Geometry check sheet. Reference: the model listing, model coordinates, mm. A direction names the side the tool comes from. Round coordinates to 2 decimals unless told otherwise and drop trailing zeros. Loops run counter-clockwise (first coordinate to the right, second up) from the corner with the lowest first, then second, coordinate; pieces in that order, holes last. Notation, with made-up numbers: (-15, -22.75) -> (36, -22.75) arc R20 ccw to (36, -2.75) -> close; hole circle Ø5 at (36.5, -26). An arc over 180 degrees is marked (long way). Use a Markdown table: item, result. Add a question column.
Q1. Gauge pin test, flat ends, axial feed: P1, Ø3, axis at y = 15, z = 1.5, coming from the -X side; P2, Ø12, axis at x = -6.5, z = 19, coming from the +Y side; P3, Ø12, axis at x = -13, z = -7, coming from the +Y side. Record the tip position at first contact, or that the pin passes through.
Q2. Material ranges on L1, parallel to X at y = 3, z = -16; L2, parallel to X at y = 3, z = -17.5; L3, parallel to Z at x = -66, y = -18, recorded low to high.
Q3. Sectioned sample at D-D, the plane x = -61.5. Enter the section's corners in (y, z).
Q4. Sectioned sample at B-B, the plane x = -71.5. Enter the section's corners in (y, z), then the cut area to 3 significant figures.
Q5. Sectioned sample at A-A, the plane z = 0. Enter the section's corners in (x, y).
Q6. Set-up check for faces 1 (the face through (-63, -22.057, 0)), 2 (the face through (-63, 14.021, 0)), 3 (the face through (-8.89, -8, -15)): record each of +Z, -Z, +X, -X, +Y, -Y from which the full face is reachable in a straight line by a thin tool's end or side.
Q7. Release check for a two-part mould opening along X. For faces 4 (the face through (-7.602, -17.576, 5.535)), 5 (the face through (-71, -18, -9.142)), 6 (the face through (-56.896, 0, -12)), 7 (the face through (-56.896, -19, 1)) record: released by +X, released by -X, zero draft, split by the parting line, or undercut.
Q8. Sectioned sample at C-C, the plane y = 0. Enter the section's corners in (x, z).
```python
from build123d import *

# Parameters (mm, degrees)
F0_R      = 24.4143154864
F1_DEPTH  = 6.35
F2_R      = 18.4271469793
F3_DEPTH  = 2.54
F4_R      = 16.7830167103
F4_R_2    = 11.3536850354
F5_DEPTH  = 48.006
F7_DEPTH  = 12.7
F9_R      = 0.7955502835
F10_DEPTH = 25.4
F11_R     = 0.6602201081
F12_DEPTH = 25.4
F14_DEPTH = 2.54
F16_DEPTH = 17.018


with BuildPart() as f1:
    # F0 (on Right) → F1 (new body, symmetric)
    with BuildSketch(Plane.YZ):
        Circle(F0_R)
    extrude(amount=F1_DEPTH, both=True)

    # F2 (on face) → F3 (join)
    with BuildSketch(Plane(origin=(-6.35, 0, 0), x_dir=(0, -1, 0), z_dir=(-1, 0, 0))):
        Circle(F2_R)
    extrude(amount=F3_DEPTH)

    # F4 (on face) → F5 (join)
    with BuildSketch(Plane(origin=(-8.89, 0, 0), x_dir=(0, -1, 0), z_dir=(-1, 0, 0))):
        Circle(F4_R)
        Circle(F4_R_2, mode=Mode.SUBTRACT)
        Circle(F4_R_2)
    extrude(amount=F5_DEPTH)

    # F6 (on face) → F7 (join)
    with BuildSketch(Plane(origin=(-56.896, 0, 0), x_dir=(0, -1, 0), z_dir=(-1, 0, 0))):
        with BuildLine():
            Line((-14.0211542356, 9.2237131244), (-14.0211542356, -9.2237131244))
            Line((-14.0211542356, -9.2237131244), (14.0211542356, -9.2237131244))
            ThreePointArc((14.0211542356, -9.2237131244), (16.0777317389, -4.814165767), (16.7830167103, 0))
            ThreePointArc((16.7830167103, 0), (15.8513574313, 5.5139928803), (13.1598161847, 10.4157999158))
            Line((13.1598161847, 10.4157999158), (-13.1598161847, 10.4157999158))
            ThreePointArc((-13.1598161847, 10.4157999158), (-13.6035493889, 9.8291959958), (-14.0211542356, 9.2237131244))
        make_face()
        with BuildLine():
            ThreePointArc((16.7830167103, 0), (16.0777317389, -4.814165767), (14.0211542356, -9.2237131244))
            Line((14.0211542356, -9.2237131244), (22.0571234822, -9.2237131244))
            Line((22.0571234822, -9.2237131244), (22.0571234822, 10.4157999158))
            Line((22.0571234822, 10.4157999158), (13.1598161847, 10.4157999158))
            ThreePointArc((13.1598161847, 10.4157999158), (15.8513574313, 5.5139928803), (16.7830167103, 0))
        make_face()
    extrude(amount=F7_DEPTH)

    # F9 (on face) → F10 (join)
    with BuildSketch(Plane(origin=(-56.896, 0, 0), x_dir=(0, -1, 0), z_dir=(-1, 0, 0))):
        with Locations((-13.1598161847, 9.6820201725)):
            Circle(F9_R)
    extrude(amount=F10_DEPTH)

    # F11 (on face) → F12 (join)
    with BuildSketch(Plane(origin=(-56.896, 0, 0), x_dir=(0, -1, 0), z_dir=(-1, 0, 0))):
        with Locations((-14.0211542356, -9.2237131244)):
            Circle(F11_R)
    extrude(amount=F12_DEPTH)

    # F13 (on face) → F14 (join)
    with BuildSketch(Plane.XY.offset(10.4157999158)):
        with BuildLine():
            Line((-69.596, -22.0571234822), (-69.596, -15.0072947145))
            ThreePointArc((-69.596, -15.0072947145), (-73.1209143839, -18.5322090983), (-69.596, -22.0571234822))
        make_face()
    extrude(amount=-F14_DEPTH)

    # F16 (add): a face of the model
    f16_faces = [f1.faces().sort_by_distance(p)[0] for p in [
        (-71.0920201285, -18.5322090983, 7.8757999158),
    ]]
    extrude(f16_faces, amount=F16_DEPTH)


solid = f1.part
```
Values:
| question | item | result |
|---|---|---|
| 1 | P1 | x = -69.6 |
| 1 | P2 | y = 20.66 |
| 1 | P3 | y = 18.24 |
| 2 | L1 | -56.9 to 6.35 |
| 2 | L2 | -8.89 to 6.35 |
| 2 | L3 | -9.22 to 10.42 |
| 3 | outline | (-22.06, -9.22) -> (13.36, -9.22) arc R0.66 ccw (long way) to (14.02, -8.56) -> (14.02, 9.22) arc R16.78 ccw to (13.9, 9.4) arc R0.8 ccw to (12.85, 10.42) -> (-22.06, 10.42) -> close |
| 4 | outline | (-21.5, -9.14) -> (-15.57, -9.14) -> (-15.57, 10.42) -> (-21.5, 10.42) -> close; circle Ø1.59 at (13.16, 9.68); circle Ø1.32 at (14.02, -9.22) |
| 4 | area | 119 mm^2 |
| 5 | outline | (-69.6, -22.06) -> (-56.9, -22.06) -> (-56.9, -16.78) -> (-8.89, -16.78) -> (-8.89, -18.43) -> (-6.35, -18.43) -> (-6.35, -24.41) -> (6.35, -24.41) -> (6.35, 24.41) -> (-6.35, 24.41) -> (-6.35, 18.43) -> (-8.89, 18.43) -> (-8.89, 16.78) -> (-56.9, 16.78) -> (-56.9, 14.02) -> (-69.6, 14.02) -> (-69.6, -15.01) arc R3.52 ccw to start |
| 6 | face 1 | +Z, -Z, -X, -Y |
| 6 | face 2 | +Z, -X, +Y |
| 6 | face 3 | none |
| 7 | face 4 | undercut |
| 7 | face 5 | zero draft |
| 7 | face 6 | released by -X |
| 7 | face 7 | undercut |
| 8 | outline | (-69.6, -9.22) -> (-56.9, -9.22) -> (-56.9, -16.78) -> (-8.89, -16.78) -> (-8.89, -18.43) -> (-6.35, -18.43) -> (-6.35, -24.41) -> (6.35, -24.41) -> (6.35, 24.41) -> (-6.35, 24.41) -> (-6.35, 18.43) -> (-8.89, 18.43) -> (-8.89, 16.78) -> (-56.9, 16.78) -> (-56.9, 10.42) -> (-69.6, 10.42) -> close |
